Verification items for the finished model (mm, model axes). A direction names the side the tool comes from. Give positions to 0.01 mm unless a question says otherwise; leave off trailing zeros. Write each loop counter-clockwise with the first axis right and the second up, starting at its lowest first coordinate (ties: lowest second). Pieces come first, ordered by that corner, then holes. Notation, with made-up numbers: (36.5, 68.5) -> (43.5, 68.5) arc R13 cw to (43.5, 89.5) -> close; hole circle Ø6 at (59.25, 2). An arc over 180 degrees is marked (long way). Answer as CSV lines item,"result". Start each with the question number.
1) Sectioned sample at B-B on y = 8.5. Record the cut outline in (x, z).
2) Sectioned sample at D-D on y = 6.7. Record the cut outline in (x, z), and give its area (3 significant figures).
3) Sectioned sample at A-A on z = 0. Record the cut outline in (x, y).
4) Gauge pin test, flat ends, axial feed: pin 1 Ø1 at (y, z) = (7, 2) entering from +X; pin 2 Ø1.8 at (x, z) = (15, 0) entering from +Y; pin 3 Ø2 at (x, z) = (7, 2) entering from +Y; pin 4 Ø1.5 at (x, z) = (-2, -2) entering from +Y. Record the tip position at first contact, or that the pin passes through.
5) Tool access check on faces 1 (the cylindrical face through (-0.15, 6.42, -1.6)), 2 (the cylindrical face through (0.15, 6.4, 1.58)), 3 (the cylindrical face through (0.15, 8.6, 1.58)), 4 (the flat face through (0, 6, 0)), 5 (the cylindrical face through (-16, 7, 0)). Record the directions out of +Z, -Z, +X, -X, +Y, -Y that give a thin tool (end or side, any length) a straight path to the whole face; none if there is none.
6) Sectioned sample at C-C on x = 5.5. Record the cut outline in (y, z), and give its area (3 significant figures).
7) Material ranges on L1, parallel to Z at x = 15, y = 7.6; L2, parallel to Z at x = 4.5, y = 7.3; L3, parallel to X at y = 7.35, z = 0.5, recorded low to high.
8) Mould release check, pull along X, two halves, no side actions. Record for faces 6 (the cylindrical face through (-0.15, 8.58, -1.6)), 7 (the flat face through (0, 9, 0)): released by +X, released by -X, zero draft, split by the parting line, or undercut.
```python
from build123d import *

# Parameters (mm, degrees)
BOSS_EXTRUDE1_DEPTH   = 15
F_1_0MM_DOWEL_HOLE1_D = 10
FILLET1_R             = 7
ESCALA1_SCALE         = 0.2


with BuildPart() as part:
    # Sketch1 → Boss-Extrude1 (new body)
    with BuildSketch(Plane(origin=(0, 0, 0), x_dir=(1, 0, 0), z_dir=(0, 1, 0))):
        with BuildLine():
            Line((57.679491924, 10), (-57.679491924, 10))
            ThreePointArc((-57.679491924, 10), (-95, 0), (-57.679491924, -10))
            Line((-57.679491924, -10), (57.679491924, -10))
            ThreePointArc((57.679491924, -10), (95, 0), (57.679491924, 10))
        make_face()
    extrude(amount=BOSS_EXTRUDE1_DEPTH)

    # Ø1.0mm Dowel Hole1 (through all)
    with Locations(Plane(origin=(0, 15, 0), x_dir=(1, 0, 0), z_dir=(0, 1, 0))):
        with Locations((-75, 0), (75, 0)):
            Hole(F_1_0MM_DOWEL_HOLE1_D / 2)

    # Fillet1
    fillet1_edges = [part.edges().sort_by_distance(p)[0] for p in [
        (95, 15, 0),
        (0, 15, -10),
        (-95, 15, 0),
        (0, 0, -10),
        (95, 0, 0),
        (0, 0, 10),
        (-95, 0, 0),
        (0, 15, 10),
        (-57.679491924, 7.5, -10),
        (57.679491924, 7.5, -10),
        (57.679491924, 7.5, 10),
        (-57.679491924, 7.5, 10),
    ]]
    fillet(fillet1_edges, radius=FILLET1_R)


with BuildPart() as part_1:
    # Escala1: scaled about (0, 7.5, 0)
    add(part.part.scale(ESCALA1_SCALE).moved(Location((0, 6, 0))))


solid = part_1.part
```
Ans:
1,outline,"(-12.15, -2.31) arc R1.73 cw to (-10.8, -1.67) -> (10.8, -1.67) arc R1.73 cw to (12.15, -2.31) arc R3.67 ccw (long way) to (12.15, 2.31) arc R1.73 cw to (10.8, 1.67) -> (-10.8, 1.67) arc R1.73 cw to (-12.15, 2.31) arc R3.67 ccw (long way) to start; hole circle Ø2 at (-15, 0); hole circle Ø2 at (15, 0)"
2,outline,"(-12.04, -2.4) arc R1.59 cw to (-10.8, -1.81) -> (10.8, -1.81) arc R1.59 cw to (12.04, -2.4) arc R3.81 ccw (long way) to (12.04, 2.4) arc R1.59 cw to (10.8, 1.81) -> (-10.8, 1.81) arc R1.59 cw to (-12.04, 2.4) arc R3.81 ccw (long way) to start; hole circle Ø2 at (-15, 0); hole circle Ø2 at (15, 0)"
2,area,"168 mm²"
3,outline,"(-19, 7.4) arc R1.4 ccw to (-17.6, 6) -> (-16, 6) -> (-16, 9) -> (-17.6, 9) arc R1.4 ccw to (-19, 7.6) -> close; (-14, 6) -> (14, 6) -> (14, 9) -> (-14, 9) -> close; (16, 6) -> (17.6, 6) arc R1.4 ccw to (19, 7.4) -> (19, 7.6) arc R1.4 ccw to (17.6, 9) -> (16, 9) -> close"
4,pin 1,"stops at x = 18.68"
4,pin 2,"passes through"
4,pin 3,"stops at y = 8.94"
4,pin 4,"stops at y = 8.84"
5,face 1,"-Z, -Y"
5,face 2,"+Z, -Y"
5,face 3,"+Z, +Y"
5,face 4,"+Z, -Z, +X, -X, -Y"
5,face 5,"+Y, -Y"
6,outline,"(6, -0.6) arc R1.4 ccw to (7.4, -2) -> (7.6, -2) arc R1.4 ccw to (9, -0.6) -> (9, 0.6) arc R1.4 ccw to (7.6, 2) -> (7.4, 2) arc R1.4 ccw to (6, 0.6) -> close"
6,area,"10.3 mm²"
7,L1,"z = -4 to -1, 1 to 4"
7,L2,"z = -2 to 2"
7,L3,"x = -18.97 to -15.87, -14.13 to 14.13, 15.87 to 18.97"
8,face 6,"undercut"
8,face 7,"zero draft"
